```python
from build123d import *

# Parameters (mm, degrees)
F0_R     = 44.451674
F0_R_2   = 38.390752
F1_DEPTH = 25.4
F2_R     = 5.08
F3_W     = 5.08
F3_H     = 23.807657


with BuildPart() as f1:
    # F0 (on Front) → F1 (new body)
    with BuildSketch(Plane.XZ):
        with Locations((0, 42.992625)):
            Circle(F0_R)
        with Locations((0, 42.992625)):
            Circle(F0_R_2, mode=Mode.SUBTRACT)
    extrude(amount=F1_DEPTH)

    # F2
    f2_edges = [f1.edges().sort_by_distance(p)[0] for p in [
        (-38.390752, -25.4, 42.992625),
        (-38.390752, 0, 42.992625),
    ]]
    fillet(f2_edges, radius=F2_R)

    # F3 (on Front) → F4 (revolve)
    with BuildSketch(Plane.XZ):
        with Locations((-2.54, -11.903828)):
            Rectangle(F3_W, F3_H)
    revolve(axis=Axis((0, 0, -11.903828), (0, 0, -1)))


solid = f1.part
```
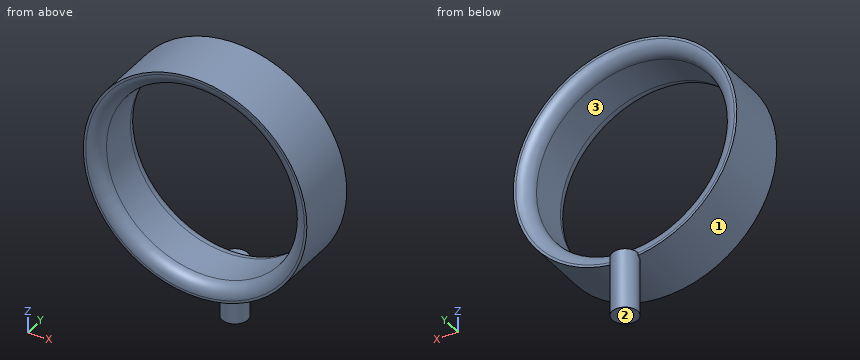
Verification items for the finished model (mm, model axes). Face numbers are marked on the shaded views. Give positions to 0.01 mm unless a question says otherwise; leave off trailing zeros. Write each loop counter-clockwise with the first axis right and the second up, starting at its lowest first coordinate (ties: lowest second). Pieces come first, ordered by that corner, then holes. Notation, with made-up numbers: M 85,77 L 111,77 A24 cw 111,114 Z; hole C 3,-35.5 d11. An arc over 180 degrees is marked long. One line per question, with ' | ' between items.
1) Gauge pin test, flat ends, axial feed: pin 1 Ø1.5 at (x, y) = (8.5, -5.5) entering from -Z; pin 2 Ø12 at (y, z) = (-17, -3.5) entering from -X; pin 3 Ø12 at (y, z) = (-13, 61) entering from -X. Record the tip position at first contact, or that the pin passes through.
Result:
pin 1: stops at z = -0.78 | pin 2: stops at x = -18.34 | pin 3: stops at x = -42.8
2) Mould release check, pull along X, two halves, no side actions. Record for the marked faces 1, 2 and 3: released by +X, released by -X, zero draft, split by the parting line, or undercut.
Result:
face 1: split by the parting line | face 2: zero draft | face 3: undercut
3) Thickness scan on line 1 along Z through (x, y) = (0, -16.75); line 2 along Z through (x, y) = (-15.5, -14.5); line 3 along Y through (x, z) = (37, 18.5). Record the ranges inside material, lowest first. Write a range as [from, to].
Result:
line 1: z = [-1.46, 4.6], [81.38, 87.44] | line 2: z = [1.33, 7.87], [78.12, 84.65] | line 3: y = [-25.4, 0]
4) Section check C-C on y = -17. Enter the section's corners in (x, z).
Result:
outline: C 0,42.99 d88.9; hole C 0,42.99 d76.78
5) Section check B-B on y = -1.5. Enter the section's corners in (x, z), plus the area to 3 significant figures.
Result:
outline: M -4.85,-23.81 L 4.85,-23.81 L 4.85,-1.19 A44.45 ccw long -4.85,-1.19 Z; hole C 0,42.99 d79.73 | area: 1,430 mm2
6) Section check A-A on x = 0. Enter the section's corners in (y, z).
Result:
outline: M -25.4,-1.46 L -5.08,-1.46 L -5.08,-23.81 L 5.08,-23.81 L 5.08,0 L -0.02,0 A5.08 ccw -5.08,4.6 L -20.32,4.6 A5.08 ccw -25.4,-0.48 Z; M -25.4,86.46 A5.08 ccw -20.32,81.38 L -5.08,81.38 A5.08 ccw 0,86.46 L 0,87.44 L -25.4,87.44 Z
